from build123d import *

# Parameters (mm, degrees)
SKETCH1_R               = 4.1
BOSS_EXTRUDE1_DEPTH     = 7
SKETCH2_R               = 6.25
BOSS_EXTRUDE2_DEPTH     = 2
SKETCH3_R               = 35
BOSS_EXTRUDE3_DEPTH     = 5
SKETCH4_R               = 25
BOSS_EXTRUDE4_DEPTH     = 5
SKETCH5_R               = 30
BOSS_EXTRUDE5_DEPTH     = 2
FILLET1_R               = 2
FILLET2_R               = 2
SKETCH6_R               = 1.5
CUT_EXTRUDE1_DEPTH      = 36
CUT_EXTRUDE1_DEPTH_BACK = 36
BOSS_EXTRUDE6_DEPTH     = 10
SKETCH9_R               = 1.75
CUT_EXTRUDE2_DEPTH      = 10
SKETCH10_R              = 52.509710967
CUT_EXTRUDE3_DEPTH      = 40


with BuildPart() as part:
    # Sketch1 → Boss-Extrude1 (new body)
    with BuildSketch(Plane.XY):
        Circle(SKETCH1_R)
    extrude(amount=BOSS_EXTRUDE1_DEPTH)

    # Sketch2 → Boss-Extrude2 (add)
    with BuildSketch(Plane.XY.offset(7)):
        Circle(SKETCH2_R)
    extrude(amount=BOSS_EXTRUDE2_DEPTH)

    # Sketch3 → Boss-Extrude3 (add)
    with BuildSketch(Plane.XY.offset(9)):
        Circle(SKETCH3_R)
    extrude(amount=BOSS_EXTRUDE3_DEPTH)

    # Sketch4 → Boss-Extrude4 (add)
    with BuildSketch(Plane.XY.offset(14)):
        Circle(SKETCH4_R)
    extrude(amount=BOSS_EXTRUDE4_DEPTH)

    # Sketch5 → Boss-Extrude5 (add)
    with BuildSketch(Plane.XY.offset(19)):
        Circle(SKETCH5_R)
    extrude(amount=BOSS_EXTRUDE5_DEPTH)

    # Fillet1
    fillet1_edges = [part.edges().sort_by_distance(p)[0] for p in [
        (-25, 0, 19),
    ]]
    fillet(fillet1_edges, radius=FILLET1_R)

    # Fillet2
    fillet2_edges = [part.edges().sort_by_distance(p)[0] for p in [
        (-25, 0, 14),
    ]]
    fillet(fillet2_edges, radius=FILLET2_R)

    # Sketch6 → Cut-Extrude1 (cut, two sides)
    with BuildSketch(Plane(origin=(0, 0, 0), x_dir=(1, 0, 0), z_dir=(0, 1, 0))) as cut_extrude1_sk:
        with Locations((0.008646323, -16.5)):
            Circle(SKETCH6_R)
    extrude(amount=CUT_EXTRUDE1_DEPTH, mode=Mode.SUBTRACT)
    extrude(cut_extrude1_sk.sketch, amount=-CUT_EXTRUDE1_DEPTH_BACK, mode=Mode.SUBTRACT)

    # Sketch7 → Boss-Extrude6 (add)
    with BuildSketch(Plane(origin=(0, 0, 9), x_dir=(-1, 0, 0), z_dir=(0, 0, -1))):
        with BuildLine():
            Line((10, -33.541019662), (10, -33.735334875))
            Line((10, -33.735334875), (10, -43.735334875))
            Line((10, -43.735334875), (-10, -43.735334875))
            Line((-10, -43.735334875), (-10, -33.735334875))
            Line((-10, -33.735334875), (-10, -33.541019662))
            ThreePointArc((-10, -33.541019662), (-28.062430401, -20.916500663), (-35, 0))
            Line((-35, 0), (-27, 0))
            ThreePointArc((-27, 0), (-15.149257408, -22.349496639), (10, -25.079872408))
            Line((10, -25.079872408), (10, -33.541019662))
        make_face()
    extrude(amount=BOSS_EXTRUDE6_DEPTH)

    # Sketch9 → Cut-Extrude2 (cut)
    with BuildSketch(Plane(origin=(0, 0, -1), x_dir=(-1, 0, 0), z_dir=(0, 0, -1))):
        with Locations((5, -38.638177269)):
            Circle(SKETCH9_R)
        with Locations((-5, -38.638177269)):
            Circle(SKETCH9_R)
    extrude(amount=-CUT_EXTRUDE2_DEPTH, mode=Mode.SUBTRACT)

    # Sketch10 → Cut-Extrude3 (cut)
    with BuildSketch(Plane.XY.offset(14)):
        Circle(SKETCH10_R)
    extrude(amount=CUT_EXTRUDE3_DEPTH, mode=Mode.SUBTRACT)


solid = part.part
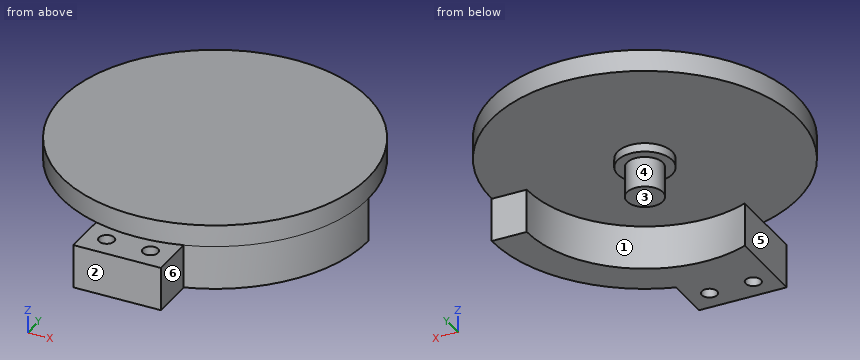
Geometry: final body of the model. Coordinates: model frame, mm. Face numbers are marked on the shaded views. A direction names the side the tool comes from. Give positions to 0.01 mm unless a question says otherwise; leave off trailing zeros. Order: outer loops, then holes, each group sorted by start corner. A loop starts at its lowest first (then second) coordinate and runs counter-clockwise, first axis right, second up. Notation, with made-up numbers: (-34.75, 13.5) - (-28.75, 13.5) arc R22 cw to (-28.75, 38.5) - close; hole circle Ø5 at (10, -22). An arc over 180 degrees is marked (long way). Use CSV: the item, a comma, the result in double quotes.
1. Contact query for flat-ended pins moving along their axis: pin 1 (4 mm diameter, centred on y = -1, z = 10, fed in from -X); pin 2 (5 mm diameter, centred on y = -40.5, z = 1.5, fed in from +X); pin 3 (2 mm diameter, centred on y = -7.5, z = 2.5, fed in from +X); pin 4 (20.5 mm diameter, centred on x = 1.5, y = -10.5, fed in from -Z). Output: stop coordinate, or through.
Answers below:
pin 1,"x = -35"
pin 2,"x = 10"
pin 3,"x = 34.39"
pin 4,"z = 0"
2. Access query for the marked faces 4, 5 and 6. Directions: +Z, -Z, +X, -X, +Y, -Y. A direction counts if a zero-diameter tool reaches every point of the face in a straight line with its end or side. Return the directions, or none.
Answers below:
face 4,"-Z"
face 5,"-Z, -X, +Y, -Y"
face 6,"+Z, -Z, +X, -Y"
3. Mould query, pull axis Y, two halves, no side actions, for the marked faces 1, 2 and 3. Classes: +Y half, -Y half, draft (parallel to the pull), parting line (faces both ways), or undercut.
Answers below:
face 1,"undercut"
face 2,"-Y half"
face 3,"draft"
4. Section query C-C (x = 20). Output: boundary loops of the cut face in (y, z), plus the area to 3 significant figures.
Answers below:
outline,"(-28.72, -1) - (-18.14, -1) - (-18.14, 9) - (28.72, 9) - (28.72, 14) - (-28.72, 14) - close"
area,"393 mm2"
5. Section query A-A (x = -5). Output: boundary loops of the cut face in (y, z).
Answers below:
outline,"(-43.74, -1) - (-40.39, -1) - (-40.39, 9) - (-43.74, 9) - close; (-36.89, -1) - (-26.53, -1) - (-26.53, 9) - (-3.75, 9) - (-3.75, 7) - (3.75, 7) - (3.75, 9) - (34.64, 9) - (34.64, 14) - (-34.64, 14) - (-34.64, 9) - (-36.89, 9) - close"
6. Section query B-B (y = -1). Output: boundary loops of the cut face in (x, z).
Answers below:
outline,"(-34.99, 9) - (-6.17, 9) - (-6.17, 7) - (-3.98, 7) - (-3.98, 0) - (3.98, 0) - (3.98, 7) - (6.17, 7) - (6.17, 9) - (26.98, 9) - (26.98, -1) - (34.99, -1) - (34.99, 14) - (-34.99, 14) - close"
7. Section query D-D (z = 10.75). Output: boundary loops of the cut face in (x, y).
Answers below:
outline,"circle Ø70 at (0, 0)"
8. Material intervals for line 1 along Z through (x, y) = (7, 9); line 2 along X through (y, z) = (-35, 5.5); line 3 along Y through (x, z) = (5, 1), sorted ascending. Write a range as from..to.
Answers below:
line 1,"9..14"
line 2,"-10..10"
line 3,"-43.74..-40.39, -36.89..-26.53"
